```python
from build123d import *

# Parameters (mm, degrees)
CROQUIS1_R              = 1.45
CROQUIS1_W              = 100
CROQUIS1_H              = 100
SALIENTE_EXTRUIR1_DEPTH = 5


with BuildPart() as part:
    # Croquis1 → Saliente-Extruir1 (new body)
    with BuildSketch(Plane(origin=(0, 0, 0), x_dir=(1, 0, 0), z_dir=(0, 1, 0))):
        Polygon((0, 0), (-14.5, 14.5), (-14.5, 132.5), (0, 147), (163, 147), (177.5, 132.5), (177.5, 14.5), (163, 0), align=None)
        with Locations(Location((18.5, 73.5, 0), (0, 0, 270))):
            Circle(CROQUIS1_R, mode=Mode.SUBTRACT)
        with Locations(Location((144.5, 73.5, 0), (0, 0, 270))):
            Circle(CROQUIS1_R, mode=Mode.SUBTRACT)
        with Locations((81.5, 73.5)):
            Rectangle(CROQUIS1_W, CROQUIS1_H, mode=Mode.SUBTRACT)
    extrude(amount=SALIENTE_EXTRUIR1_DEPTH)


solid = part.part
```
Build history of the part. All positions in model axes, mm. A direction names the side the tool comes from. Round coordinates to 2 decimals unless told otherwise and drop trailing zeros. Write each loop counter-clockwise with the first axis right and the second up, starting at its lowest first coordinate (ties: lowest second). Pieces come first, ordered by that corner, then holes.
1) Band-saw the part on A-A, the plane x = 89. List the corners of the cut face in (y, z).
2) Drill centre lines: probe 1 along X at (y, z) = (2, -73.5); probe 2 along X at (y, z) = (2.8, -63); probe 3 along Z at (x, y) = (60.5, 3.65). Where is each one in solid material? Low to high.
3) Band-saw the part on C-C, the plane y = 3.65. List the corners of the cut face in (x, z).
4) Pin check, flat tip, straight feed: pin 1 (2.5 mm diameter, centred on x = 144.5, z = -73.5, fed in from +Y). Stop position of the tip, or through.
5) Band-saw the part on D-D, the plane z = -138. List the corners of the cut face in (x, y).
6) 3-axis set-ups, long thin cutter, end or side, ignore diameter. For faces 4 (the flat face through (170, 2, -140)), 5 (the flat face through (131.5, 2, -73)): which of +Z, -Z, +X, -X, +Y, -Y reach the whole face in a straight line?
7) Band-saw the part on B-B, the plane z = -61. List the corners of the cut face in (x, y).
8) Mould opens along Z. For faces 1 (the flat face through (81, 2, -123.5)), 2 (the flat face through (-14.5, 2, -73)), 3 (the flat face through (-7, 2, -7)) say: +Z half, -Z half, draft (parallel to the pull), parting line (faces both ways), or undercut.
Ans:
1. outline: (0, -147) - (5, -147) - (5, -123.5) - (0, -123.5) - close; (0, -23.5) - (5, -23.5) - (5, 0) - (0, 0) - close
2. probe 1: x = -14.5 to 17.05, 19.95 to 31.5, 131.5 to 143.05, 145.95 to 177.5
2. probe 2: x = -14.5 to 31.5, 131.5 to 177.5
2. probe 3: z = -147 to -123.5, -23.5 to 0
3. outline: (-14.5, -132.5) - (0, -147) - (163, -147) - (177.5, -132.5) - (177.5, -14.5) - (163, 0) - (0, 0) - (-14.5, -14.5) - close; hole circle Ø2.9 at (18.5, -73.5); hole (31.5, -123.5) - (131.5, -123.5) - (131.5, -23.5) - (31.5, -23.5) - close; hole circle Ø2.9 at (144.5, -73.5)
4. pin 1: passes through
5. outline: (-9, 0) - (172, 0) - (172, 5) - (-9, 5) - close
6. face 4: -Z, +X, +Y, -Y
6. face 5: +Y, -Y
7. outline: (-14.5, 0) - (31.5, 0) - (31.5, 5) - (-14.5, 5) - close; (131.5, 0) - (177.5, 0) - (177.5, 5) - (131.5, 5) - close
8. face 1: undercut
8. face 2: draft
8. face 3: +Z half
